Part model, mm, in its own coordinate system. Face numbers are marked on the shaded views. A direction names the side the tool comes from. Give positions to 0.01 mm unless a question says otherwise; leave off trailing zeros. Write each loop counter-clockwise with the first axis right and the second up, starting at its lowest first coordinate (ties: lowest second). Pieces come first, ordered by that corner, then holes. Notation, with made-up numbers: M 52.5,88.25 L 95.5,88.25 A10 ccw 95.5,95.25 Z; hole C 13.25,71.25 d5. An arc over 180 degrees is marked long. Answer as CSV lines item,"result". Start each with the question number.
1) Tool access for the marked faces 1 and 2: list every direction of +Z, -Z, +X, -X, +Y, -Y with a clear straight run to the whole face (end or side of a thin tool).
2) Slice it at B-B, the plane y = -144. Give the cut face in (x, z), plus the area to 3 significant figures.
3) Mould opens along X. For the marked faces 3, 4 and 5 say: pulls with the +X half, pulls with the -X half, needs draft (parallel to the pull), parting line crosses it, or undercut.
4) Slice it at A-A, the plane z = 57.5. Give the cut face in (x, y), plus the area to 4 significant figures.
5) Pin check, flat tips, straight feed: pin 1 Ø2 at (y, z) = (86.5, 69.5) entering from +X; pin 2 Ø1.2 at (y, z) = (18.5, 68.5) entering from -X; pin 3 Ø3 at (x, z) = (-103.5, 69) entering from -Y. Stop position of each tip, or through.
6) Wall check: line 1 along Y through (x, z) = (-191, 8); line 2 along X through (y, z) = (94.5, 28.5); line 3 along Z through (x, y) = (114.5, 51). Give the ranges that are in metal, low to high. Write a range as from..to.
7) Slice it at C-C, the plane x = -104. Give the cut face in (y, z).
```python
from build123d import *

# Parameters (mm, degrees)
F0_W     = 550
F0_H     = 505
F1_DEPTH = 5
F2_W     = 540
F2_H     = 495
F3_DEPTH = 61.5
F5_DEPTH = 4
F7_DEPTH = 25.4


with BuildPart() as f1:
    # F0 (on Top) → F1 (new body)
    with BuildSketch(Plane.XY):
        Rectangle(F0_W, F0_H)
    extrude(amount=F1_DEPTH)

    # F2 (on face) → F3 (join)
    with BuildSketch(Plane.XY.offset(5)):
        Polygon((-270, -252.5), (275, -252.5), (275, 247.5), (275, 252.5), (270, 252.5), (-275, 252.5), (-275, -247.5), (-275, -252.5), align=None)
        Rectangle(F2_W, F2_H, mode=Mode.SUBTRACT)
    extrude(amount=F3_DEPTH)

    # F4 (on face) → F5 (join)
    with BuildSketch(Plane.XY.offset(66.5)):
        Polygon((273, 250.5), (271, 250.5), (-273, 250.5), (-273, -248.5), (-273, -250.5), (273, -250.5), (273, 248.5), align=None)
        Polygon((-271, -248.5), (-271, -247.5), (-271, 248.5), (270, 248.5), (271, 248.5), (271, 247.5), (271, -248.5), (-270, -248.5), align=None, mode=Mode.SUBTRACT)
    extrude(amount=F5_DEPTH)

    # F6 (on face) → F7 (cut)
    with BuildSketch(Plane.XZ.offset(250.5)):
        with BuildLine():
            Line((4.5, 70.5), (3.5, 70.5))
            Line((3.5, 70.5), (3.5, 69.5))
            ThreePointArc((3.5, 69.5), (4.5, 68.5), (5.5, 69.5))
            Line((5.5, 69.5), (5.5, 70.5))
            Line((5.5, 70.5), (4.5, 70.5))
        make_face()
        with BuildLine():
            Line((1.5, 70.5), (0.5, 70.5))
            Line((0.5, 70.5), (0.5, 69.5))
            ThreePointArc((0.5, 69.5), (1.5, 68.5), (2.5, 69.5))
            Line((2.5, 69.5), (2.5, 70.5))
            Line((2.5, 70.5), (1.5, 70.5))
        make_face()
        with BuildLine():
            Line((-3.5, 69.5), (-3.5, 70.5))
            Line((-3.5, 70.5), (-4.5, 70.5))
            Line((-4.5, 70.5), (-5.5, 70.5))
            Line((-5.5, 70.5), (-5.5, 69.5))
            ThreePointArc((-5.5, 69.5), (-4.5, 68.5), (-3.5, 69.5))
        make_face()
        with BuildLine():
            Line((-0.5, 69.5), (-0.5, 70.5))
            Line((-0.5, 70.5), (-1.5, 70.5))
            Line((-1.5, 70.5), (-2.5, 70.5))
            Line((-2.5, 70.5), (-2.5, 69.5))
            ThreePointArc((-2.5, 69.5), (-1.5, 68.5), (-0.5, 69.5))
        make_face()
    extrude(amount=-F7_DEPTH, mode=Mode.SUBTRACT)


solid = f1.part
```
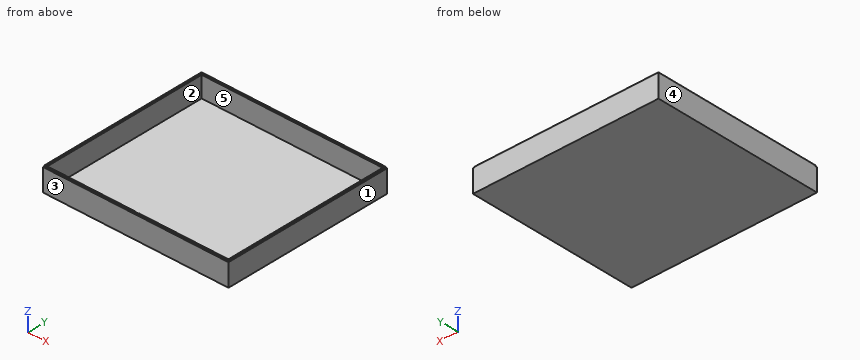
Found:
1,face 1,"+Z, -Z, +X, +Y, -Y"
1,face 2,"+Z"
2,outline,"M -275,0 L 275,0 L 275,66.5 L 273,66.5 L 273,70.5 L 271,70.5 L 271,66.5 L 270,66.5 L 270,5 L -270,5 L -270,66.5 L -271,66.5 L -271,70.5 L -273,70.5 L -273,66.5 L -275,66.5 Z"
2,area,"3,380 mm²"
3,face 3,"needs draft"
3,face 4,"pulls with the -X half"
3,face 5,"undercut"
4,outline,"M -275,-252.5 L 275,-252.5 L 275,252.5 L -275,252.5 Z; hole M -270,-247.5 L 270,-247.5 L 270,247.5 L -270,247.5 Z"
4,area,"10,450 mm²"
5,pin 1,"x = 273"
5,pin 2,"x = -273"
5,pin 3,"y = -250.5"
6,line 1,"-252.5..-247.5, 247.5..252.5"
6,line 2,"-275..-270, 270..275"
6,line 3,"0..5"
7,outline,"M -252.5,0 L 252.5,0 L 252.5,66.5 L 250.5,66.5 L 250.5,70.5 L 248.5,70.5 L 248.5,66.5 L 247.5,66.5 L 247.5,5 L -247.5,5 L -247.5,66.5 L -248.5,66.5 L -248.5,70.5 L -250.5,70.5 L -250.5,66.5 L -252.5,66.5 Z"
